Work out the finished part from the listing and answer in its coordinate system (mm). A direction names the side the tool comes from. Round coordinates to 2 decimals unless told otherwise and drop trailing zeros. Loops run counter-clockwise (first coordinate to the right, second up) from the corner with the lowest first, then second, coordinate; pieces in that order, holes last. Notation, with made-up numbers: (7, -24) - (37, -24) arc R9 ccw to (37, -14) - close; hole circle Ø6 at (76.25, -23). An arc over 180 degrees is marked (long way). Return JSON: item names as keys, results as strings.
from build123d import *

# Parameters (mm, degrees)
BOSS_EXTRUDE1_DEPTH = 3
CUT_EXTRUDE1_DEPTH  = 1.5
SKETCH4_W           = 10
SKETCH4_H           = 3
BOSS_EXTRUDE3_DEPTH = 10


with BuildPart() as part:
    # Sketch1 → Boss-Extrude1 (new body)
    with BuildSketch(Plane(origin=(0, 0, 0), x_dir=(1, 0, 0), z_dir=(0, 1, 0))):
        with BuildLine():
            Line((-7.499999551, 0), (22.5, 0))
            ThreePointArc((22.5, 0), (25, 2.5), (22.5, 5))
            Line((22.5, 5), (-7.5, 5))
            ThreePointArc((-7.5, 5), (-10, 2.499999775), (-7.499999551, 0))
        make_face()
    extrude(amount=BOSS_EXTRUDE1_DEPTH)

    # Sketch2 → Cut-Extrude1 (cut)
    with BuildSketch(Plane.XZ):
        with BuildLine():
            Line((-7.5, -4), (22.5, -4))
            ThreePointArc((22.5, -4), (24, -2.5), (22.5, -1))
            Line((22.5, -1), (-7.49999973, -1))
            ThreePointArc((-7.49999973, -1), (-9, -2.499999865), (-7.5, -4))
        make_face()
    extrude(amount=-CUT_EXTRUDE1_DEPTH, mode=Mode.SUBTRACT)

    # Sketch4 → Boss-Extrude3 (add)
    with BuildSketch(Plane(origin=(0, 0, -5), x_dir=(-1, 0, 0), z_dir=(0, 0, -1))):
        with Locations((-7.5, 1.5)):
            Rectangle(SKETCH4_W, SKETCH4_H)
    extrude(amount=BOSS_EXTRUDE3_DEPTH)


solid = part.part
1) Section C-C (y = 0.8) is taken. Give the vertices of the cut face in (x, z), and give its area (3 significant figures).
Verdict:
{"outline": "(-7.5, -5) - (2.5, -5) - (2.5, -15) - (12.5, -15) - (12.5, -5) - (22.5, -5) arc R2.5 ccw to (22.5, 0) - (-7.5, 0) arc R2.5 ccw to start; hole (-7.5, -4) - (22.5, -4) arc R1.5 ccw to (22.5, -1) - (-7.5, -1) arc R1.5 ccw to start", "area": "173 mm2"}
2) Find the intervals of material crossed by L1, parallel to Z at x = -0.5, y = 0.4; L2, parallel to Z at x = 3, y = 0.9; L3, parallel to X at y = 1.6, z = -6.25, in increasing order.
Verdict:
{"L1": "z = -5 to -4, -1 to 0", "L2": "z = -15 to -4, -1 to 0", "L3": "x = 2.5 to 12.5"}
3) A tool of negligible diameter and unlimited length cuts with its end or side. For faces 5 (the flat face through (-2, 1, -5)), 6 (the flat face through (8, 1, -1)), 7 (the flat face through (12.5, 1, -10)), from which of +Z, -Z, +X, -X, +Y, -Y can it reach the whole face along a straight path? Write none if from no direction.
Verdict:
{"face 5": "-Z, -X, +Y, -Y", "face 6": "-Y", "face 7": "-Z, +X, +Y, -Y"}
4) Flat-ended cylindrical pins translate along their axes: pin 1 (1.5 mm diameter, centred on x = -0.5, y = 1.5, fed in from -Z); pin 2 (1.5 mm diameter, centred on x = -0.5, z = -2.5, fed in from -Y). Find the tip coordinate at first contact, or state that the pin passes through.
Verdict:
{"pin 1": "stops at z = -5", "pin 2": "stops at y = 1.5"}
5) Section A-A (y = 2.3) is taken. Give the vertices of the cut face in (x, z), and give its area (3 significant figures).
Verdict:
{"outline": "(-7.5, -5) - (2.5, -5) - (2.5, -15) - (12.5, -15) - (12.5, -5) - (22.5, -5) arc R2.5 ccw to (22.5, 0) - (-7.5, 0) arc R2.5 ccw to start", "area": "270 mm2"}
6) Section B-B (z = -2.5) is taken. Give the vertices of the cut face in (x, y).
Verdict:
{"outline": "(-10, 0) - (-9, 0) - (-9, 1.5) - (24, 1.5) - (24, 0) - (25, 0) - (25, 3) - (-10, 3) - close"}
7) Determine the mould class of faces 1 (the cylindrical face through (-9, 0.7, -2.5)), 2 (the cylindrical face through (24, 0.7, -2.5)), 3 (the cylindrical face through (25, 1.5, -2.4)), 4 (the flat face through (2.5, 1, -10)) for opening direction Z: pulls with the +Z half, pulls with the -Z half, needs draft (parallel to the pull), parting line crosses it, or undercut.
Verdict:
{"face 1": "undercut", "face 2": "undercut", "face 3": "parting line crosses it", "face 4": "needs draft"}
